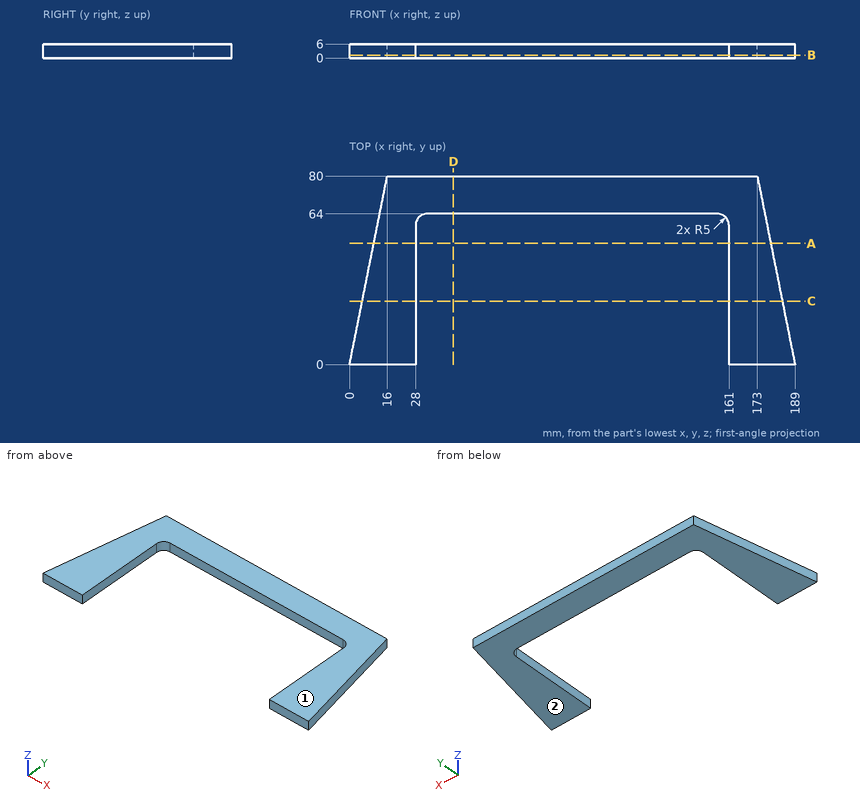
Study the drawing (mm; zero at the part's minimum x, y, z) and answer. Coordinates: 2 decimals unless noted, no trailing zeros. Order: outer loops, then holes, each group sorted by start corner. A loop starts at its lowest first (then second) coordinate and runs counter-clockwise, first axis right, second up. Notation, with made-up numbers: M -5.75,-7 L 49.25,-7 A17 cw 49.25,19 Z; hole C -33.75,-8 d1. An arc over 180 degrees is marked long. Answer as a JSON object with one key per item and string values. Group by question number.
1. Section D-D on x = 44 is taken. Write down the section's boundary in (y, z).
2. Straight lines are drawn through the part: line 1 (X direction, y = 50.5, z = 2); line 2 (Y direction, x = 114.5, z = 5.55); line 3 (X direction, y = 6, z = 3.5). For each, find the intervals that lie inside material, in ascending order.
3. A flat-ended cylindrical pin translates along its axis: P1, Ø3, axis at x = 69.5, z = 3.5, coming from the -Y side. Find the tip coordinate at first contact, or state that the pin passes through.
4. Section B-B on z = 1.3 is taken. Write down the section's boundary in (x, y), then the cut area to 3 significant figures.
5. Section C-C on y = 27 is taken. Write down the section's boundary in (x, z), then the cut area to 3 significant figures.
6. Determine the mould class of the marked faces 1 and 2 for opening direction Z: released by +Z, released by -Z, zero draft, split by the parting line, or undercut.
7. Section A-A on y = 51.5 is taken. Write down the section's boundary in (x, z).
Values follow:
{
 "1": {"outline": "M 64,0 L 80,0 L 80,6 L 64,6 Z"},
 "2": {"line 1": "10.1 to 28, 161 to 178.9", "line 2": "64 to 80", "line 3": "1.2 to 28, 161 to 187.8"},
 "3": {"P1": "y = 64"},
 "4": {"outline": "M 0,0 L 28,0 L 28,59 A5 cw 33,64 L 156,64 A5 cw 161,59 L 161,0 L 189,0 L 173,80 L 16,80 Z", "area": "5,340 mm2"},
 "5": {"outline": "M 5.4,0 L 28,0 L 28,6 L 5.4,6 Z; M 161,0 L 183.6,0 L 183.6,6 L 161,6 Z", "area": "271 mm2"},
 "6": {"face 1": "released by +Z", "face 2": "released by -Z"},
 "7": {"outline": "M 10.3,0 L 28,0 L 28,6 L 10.3,6 Z; M 161,0 L 178.7,0 L 178.7,6 L 161,6 Z"}
}
